CAD build for the part. Positions are in the model's coordinates, mm. Face numbers are marked on the shaded views. A direction names the side the tool comes from. Give positions to 0.01 mm unless a question says otherwise; leave off trailing zeros. Write each loop counter-clockwise with the first axis right and the second up, starting at its lowest first coordinate (ties: lowest second). Pieces come first, ordered by that corner, then holes. Notation, with made-up numbers: (47.25, 70) - (59.25, 70) arc R18 ccw to (59.25, 85) - close; hole circle Ø8 at (8.5, 44.5). An arc over 180 degrees is marked (long way). Put each result on its own line as item: value. Start each with the question number.
1. Cut at A-A on y = 2.5. List the corners of the cut face in (x, z).
2. Drop flat-ended pins along their axis: pin 1 (1 mm diameter, centred on x = 1, z = 1, fed in from -Y); pin 2 (1 mm diameter, centred on x = 2, y = 2.5, fed in from -Z); pin 3 (1.5 mm diameter, centred on x = 0, z = 0, fed in from -Y); pin 4 (2 mm diameter, centred on x = -1.5, z = -2, fed in from +Y). Give the stop position or say it passes through.
3. Cut at C-C on z = 0. List the corners of the cut face in (x, y).
4. Cut at D-D on y = 6.25. List the corners of the cut face in (x, z).
5. Cut at B-B on x = 0. List the corners of the cut face in (y, z).
6. Mould opens along Z. For the marked faces 1, 2, 3 and 4 say: +Z half, -Z half, draft (parallel to the pull), parting line (faces both ways), or undercut.
7. Wall check: line 1 (Y direction, x = 1.85, z = 1.6); line 2 (Y direction, x = 0.2, z = 0.55); line 3 (Z direction, x = -0.3, y = 0.5). Give the ranges that are in metal, low to high.
8. Tool access for the marked faces 5 and 6: list every direction of +Z, -Z, +X, -X, +Y, -Y with a clear straight run to the whole face (end or side of a thin tool).
from build123d import *

# Parameters (mm, degrees)
SALIENTE_EXTRUIR1_DEPTH = 6
CROQUIS_CARA_R          = 1.25
SALIENTE_EXTRUIR2_DEPTH = 3
REDONDEO1_R             = 0.2
CROQUIS1_R              = 1.25
CORTAR_EXTRUIR1_DEPTH   = 3


with BuildPart() as part:
    # Croquis base → Saliente-Extruir1 (new body)
    with BuildSketch(Plane(origin=(0, 0, 0), x_dir=(1, 0, 0), z_dir=(0, 1, 0))):
        Polygon((2.082277712, -1.648469855), (2.468755628, 0.979070469), (0.386477916, 2.627540324), (-2.082277712, 1.648469855), (-2.468755628, -0.979070469), (-0.386477916, -2.627540324), align=None)
    extrude(amount=SALIENTE_EXTRUIR1_DEPTH)

    # Croquis cara → Saliente-Extruir2 (add)
    with BuildSketch(Plane(origin=(0, 6, 0), x_dir=(1, 0, 0), z_dir=(0, 1, 0))):
        with Locations(Location((0, 0, 0), (0, 0, 270))):
            Circle(CROQUIS_CARA_R)
    extrude(amount=SALIENTE_EXTRUIR2_DEPTH)

    # Redondeo1
    redondeo1_edges = [part.edges().sort_by_distance(p)[0] for p in [
        (0, 9, -1.25),
    ]]
    fillet(redondeo1_edges, radius=REDONDEO1_R)

    # Croquis1 → Cortar-Extruir1 (cut)
    with BuildSketch(Plane.XZ):
        with Locations(Location((0, 0, 0), (0, 0, 90))):
            Circle(CROQUIS1_R)
    extrude(amount=-CORTAR_EXTRUIR1_DEPTH, mode=Mode.SUBTRACT)


solid = part.part
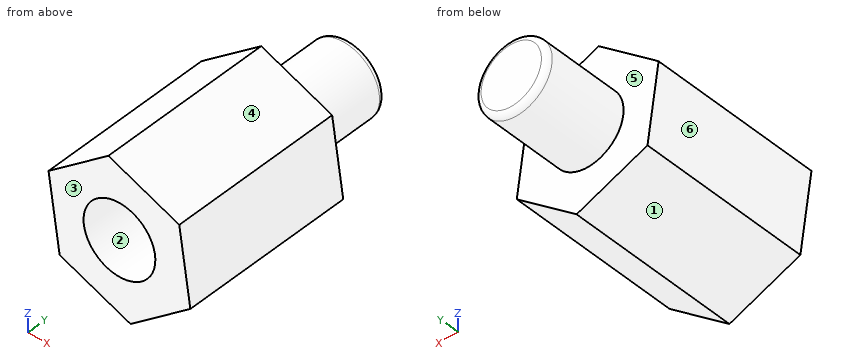
Report:
1. outline: (-2.47, 0.98) - (-2.08, -1.65) - (0.39, -2.63) - (2.47, -0.98) - (2.08, 1.65) - (-0.39, 2.63) - close; hole circle Ø2.5 at (0, 0)
2. pin 1: stops at y = 0
2. pin 2: stops at z = -1.75
2. pin 3: stops at y = 3
2. pin 4: stops at y = 6
3. outline: (-2.32, 0) - (-1.25, 0) - (-1.25, 3) - (1.25, 3) - (1.25, 0) - (2.32, 0) - (2.32, 6) - (1.25, 6) - (1.25, 8.8) arc R0.2 ccw to (1.05, 9) - (-1.05, 9) arc R0.2 ccw to (-1.25, 8.8) - (-1.25, 6) - (-2.32, 6) - close
4. outline: circle Ø2.5 at (0, 0)
5. outline: (0, -2.47) - (6, -2.47) - (6, -1.25) - (8.8, -1.25) arc R0.2 ccw to (9, -1.05) - (9, 1.05) arc R0.2 ccw to (8.8, 1.25) - (6, 1.25) - (6, 2.47) - (0, 2.47) - (0, 1.25) - (3, 1.25) - (3, -1.25) - (0, -1.25) - close
6. face 1: -Z half
6. face 2: undercut
6. face 3: draft
6. face 4: +Z half
7. line 1: y = 0 to 6
7. line 2: y = 3 to 9
7. line 3: z = -2.36 to -1.21, 1.21 to 2.59
8. face 5: +Y
8. face 6: -Z, -X, +Y, -Y
